```python
from build123d import *

# Parameters (mm, degrees)
IZIM1_R                     = 15
Y_KSEKLIK_EKSTR_ZYON2_DEPTH = 20
IZIM2_R                     = 10
KES_EKSTR_ZYON1_DEPTH       = 1
IZIM3_R                     = 10
KES_EKSTR_ZYON2_DEPTH       = 3
IZIM4_W                     = 4
IZIM4_H                     = 4
Y_KSEKLIK_EKSTR_ZYON3_DEPTH = 7
KES_EKSTR_ZYON3_DEPTH       = 7
RADYUS1_R                   = 0.15
Y_KSEKLIK_EKSTR_ZYON4_START = -0.5
IZIM6_R                     = 15.636710187
Y_KSEKLIK_EKSTR_ZYON4_DEPTH = 1


with BuildPart() as part:
    # Çizim1 → Yükseklik-Ekstrüzyon2 (new body)
    with BuildSketch(Plane(origin=(0, 0, 0), x_dir=(1, 0, 0), z_dir=(0, 1, 0))):
        Circle(IZIM1_R)
    extrude(amount=Y_KSEKLIK_EKSTR_ZYON2_DEPTH)

    # Çizim2 → Kes-Ekstrüzyon1 (cut)
    with BuildSketch(Plane(origin=(0, 20, 0), x_dir=(1, 0, 0), z_dir=(0, 1, 0))):
        Circle(IZIM2_R)
    extrude(amount=-KES_EKSTR_ZYON1_DEPTH, mode=Mode.SUBTRACT)

    # Çizim3 → Kes-Ekstrüzyon2 (cut)
    with BuildSketch(Plane.XZ):
        Circle(IZIM3_R)
    extrude(amount=-KES_EKSTR_ZYON2_DEPTH, mode=Mode.SUBTRACT)

    # Çizim4 → Yükseklik-Ekstrüzyon3 (add)
    with BuildSketch(Plane.XZ.offset(-3)):
        Rectangle(IZIM4_W, IZIM4_H)
    extrude(amount=Y_KSEKLIK_EKSTR_ZYON3_DEPTH)

    # Çizim5 → Kes-Ekstrüzyon3 (cut)
    with BuildSketch(Plane(origin=(2, 0, 0), x_dir=(0, 0, -1), z_dir=(1, 0, 0))):
        with BuildLine():
            ThreePointArc((1.060660172, -0.939339828), (-1.060660172, -0.939339828), (-1.060660172, -3.060660172))
            Line((-1.060660172, -3.060660172), (1.060660172, -0.939339828))
        make_face()
        with BuildLine():
            Line((1.060660172, -0.939339828), (-1.060660172, -3.060660172))
            ThreePointArc((-1.060660172, -3.060660172), (0.574025149, -3.385819299), (1.5, -2))
            ThreePointArc((1.5, -2), (1.385819299, -1.425974851), (1.060660172, -0.939339828))
        make_face()
    extrude(amount=-KES_EKSTR_ZYON3_DEPTH, mode=Mode.SUBTRACT)

    # Radyus1
    radyus1_edges = [part.edges().sort_by_distance(p)[0] for p in [
        (-10, 0, 0),
        (0, -4, 2),
        (0, -4, -2),
        (-15, 0, 0),
        (-15, 20, 0),
        (-10, 20, 0),
    ]]
    fillet(radyus1_edges, radius=RADYUS1_R)

    # Çizim6 → Yükseklik-Ekstrüzyon4 (add)
    with BuildSketch(Plane(origin=(0, 20, 0), x_dir=(1, 0, 0), z_dir=(0, 1, 0)).offset(Y_KSEKLIK_EKSTR_ZYON4_START)):
        Circle(IZIM6_R)
    extrude(amount=-Y_KSEKLIK_EKSTR_ZYON4_DEPTH)


solid = part.part
```
Verification items for the finished model (mm, model axes). A direction names the side the tool comes from. Give positions to 0.01 mm unless a question says otherwise; leave off trailing zeros. Order: outer loops, then holes, each group sorted by start corner. A loop starts at its lowest first (then second) coordinate and runs counter-clockwise, first axis right, second up. Notation, with made-up numbers: M 3,27.25 L 36,27.25 A13 ccw 36,32.25 Z; hole C 85,27.25 d5. An arc over 180 degrees is marked long. Answer in a Markdown table with one row per item. Add a question column.
Item 1: Gauge pin test, flat ends, axial feed: pin 1 (4.5 mm diameter, centred on y = 1, z = -0.5, fed in from +X); pin 2 (4.5 mm diameter, centred on x = 1, y = -1, fed in from -Z); pin 3 (3 mm diameter, centred on x = -7.5, y = 12, fed in from +Z); pin 4 (1.2 mm diameter, centred on y = -1.5, z = 0.5, fed in from -X). Record the tip position at first contact, or that the pin passes through.
Item 2: Scan lines: probe 1 along Z at (x, y) = (0, 1.95); probe 2 along Z at (x, y) = (0, 19.6). Record each from-to range of solid material in increasing order. Write a range as from..to.
Item 3: Tool access check on faces 4 (the flat face through (-2, 0, 0)), 5 (the flat face through (3, 20, 10)), 6 (the cylindrical face through (-2.17, 19.68, 9.76)). Record the directions out of +Z, -Z, +X, -X, +Y, -Y that give a thin tool (end or side, any length) a straight path to the whole face; none if there is none.
Item 4: Mould release check, pull along Z, two halves, no side actions. Record for faces 1 (the flat face through (13, 18.5, 8)), 2 (the cylindrical face through (14.444, 19.007, 5.989)), 3 (the flat face through (2, 0, 0)): released by +Z, released by -Z, zero draft, split by the parting line, or undercut.
Item 5: Section check A-A, the plane y = -2.5. Enter the section's corners in (x, z).
Item 6: Section check B-B, the plane y = 4.25. Enter the section's corners in (x, z), and give its area (3 significant figures).
Filled sheet:
| question | item | result |
|---|---|---|
| 1 | pin 1 | stops at x = 15 |
| 1 | pin 2 | stops at z = -15 |
| 1 | pin 3 | stops at z = 13.75 |
| 1 | pin 4 | passes through |
| 2 | probe 1 | z = -15..-10, -2..2, 10..15 |
| 2 | probe 2 | z = -15..-10, 10..15 |
| 3 | face 4 | -Y |
| 3 | face 5 | +Z, -Z, +X, -X, +Y |
| 3 | face 6 | +Y |
| 4 | face 1 | zero draft |
| 4 | face 2 | split by the parting line |
| 4 | face 3 | undercut |
| 5 | outline | M -2,-2 L 2,-2 L 2,-1.41 L -2,-1.41 Z; M -2,1.41 L 2,1.41 L 2,2 L -2,2 Z |
| 6 | outline | C 0,0 d30 |
| 6 | area | 707 mm^2 |
